from build123d import *

# Parameters (mm, degrees)
F0_W         = 34.925
F0_H         = 52.705
F1_DEPTH     = 9.7155
F2_W         = 25.781
F2_H         = 43.18
F2_H_2       = 40.005
F3_DEPTH     = 25.4
F4_R         = 8.255
F5_SIZE      = 0.8255
F6_R         = 1.5875
F7_DEPTH     = 25.4
F8_T1_DEPTH  = 34.1927991577
F9_SIZE      = 0.79375
F10_R        = 1.5875
F11_DEPTH    = 25.4
F13_R        = 7.493
F14_DEPTH    = 50.8
F15_T1_DEPTH = 13.2391086204
F15_T3_DEPTH = 13.2391086204
F16_W        = 2.54
F16_H        = 15.24
F17_DEPTH    = 25.4


# Not quite as in the source:
# - a fillet or chamfer that OpenCascade refuses, or shapes differently, is made with other operations: its cross-section is extruded or revolved along the edge and cut away or added
# - a feature names something its author has since deleted; it is built from what else it names


with BuildPart() as f1:
    # F0 (on Top) → F1 (new body)
    with BuildSketch(Plane.XY):
        with Locations((-17.4625, -26.3525)):
            Rectangle(F0_W, F0_H)
        with Locations((-17.4625, 26.3525)):
            Rectangle(F0_W, F0_H)
        Polygon((0, 52.705), (0, 0), (0, -52.705), (34.925, -52.705), (34.925, 0), (34.925, 52.705), align=None)
    extrude(amount=F1_DEPTH)

    # F2 (on face) → F3 (cut)
    with BuildSketch(Plane.XY.offset(9.7155)):
        with Locations((-12.8905, -21.59)):
            Rectangle(F2_W, F2_H)
        with Locations((-12.8905, 20.0025)):
            Rectangle(F2_W, F2_H_2)
        with Locations((12.8905, -21.59)):
            Rectangle(F2_W, F2_H)
        with Locations((12.8905, 20.0025)):
            Rectangle(F2_W, F2_H_2)
    extrude(amount=-F3_DEPTH, mode=Mode.SUBTRACT)

    # F4
    f4_edges = [f1.edges().sort_by_distance(p)[0] for p in [
        (-25.781, 40.005, 4.85775),
        (25.781, 40.005, 4.85775),
        (-25.781, -43.18, 4.85775),
        (25.781, -43.18, 4.85775),
    ]]
    fillet(f4_edges, radius=F4_R)

    # F5
    f5_edges = [f1.edges().sort_by_distance(p)[0] for p in [
        (-34.925, 0, 9.7155),
        (-25.781, -1.5875, 9.7155),
        (34.925, 0, 9.7155),
        (0, -52.705, 9.7155),
        (0, 52.705, 9.7155),
        (-34.925, 0, 0),
        (0, -52.705, 0),
        (34.925, 0, 0),
        (25.781, -1.5875, 0),
        (0, 52.705, 0),
        (-25.781, -1.5875, 0),
        (-23.363166, 37.587166, 0),
        (-23.363166, -40.762166, 0),
        (0, 40.005, 0),
        (0, -43.18, 0),
        (23.363166, 37.587166, 0),
        (23.363166, -40.762166, 0),
        (-23.363166, 37.587166, 9.7155),
        (-23.363166, -40.762166, 9.7155),
        (0, 40.005, 9.7155),
        (0, -43.18, 9.7155),
        (23.363166, 37.587166, 9.7155),
        (23.363166, -40.762166, 9.7155),
        (25.781, -1.5875, 9.7155),
    ]]
    chamfer(f5_edges, length=F5_SIZE)

    # F6 (on face) → F7 (cut)
    with BuildSketch(Plane(origin=(0, 52.705, 0), x_dir=(-1, 0, 0), z_dir=(0, 1, 0))):
        with Locations((-16.51, 4.7625)):
            Circle(F6_R)
        with Locations((16.51, 4.7625)):
            Circle(F6_R)
    extrude(amount=-F7_DEPTH, mode=Mode.SUBTRACT)

    # F8: chamfer of 5.08 on 2 edges, made by hand

    # F8_s2 → F8_t1 (cut)
    with BuildSketch(Plane.XY.offset(-12.2386495789)):
        Polygon((-34.925, -47.625), (-29.845, -52.705), (-34.925, -52.705), align=None)
        Polygon((29.845, -52.705), (34.925, -47.625), (34.925, -52.705), align=None)
    extrude(amount=F8_T1_DEPTH, mode=Mode.SUBTRACT)

    # F9
    f9_edges = [f1.edges().sort_by_distance(p)[0] for p in [
        (-32.385, -50.165, 0),
        (32.385, -50.165, 0),
        (32.385, -50.165, 9.7155),
        (-32.385, -50.165, 9.7155),
    ]]
    chamfer(f9_edges, length=F9_SIZE)

    # F10 (on face) → F11 (cut)
    with BuildSketch(Plane.XZ.offset(52.705)):
        with Locations((0, 4.7625)):
            Circle(F10_R)
    extrude(amount=-F11_DEPTH, mode=Mode.SUBTRACT)

    # F13 (on face) + F2 (on face) → F14 (cut)
    with BuildSketch(Plane(origin=(8.524875, 0, -14.7655166282), x_dir=(0.8660254038, 0, 0.5), z_dir=(0.5, 0, -0.8660254038))):
        with Locations((2.460086914, -52.705)):
            Circle(F13_R)
    with BuildSketch(Plane.XY.offset(9.7155)):
        with Locations((-12.8905, -21.59)):
            Rectangle(F2_W, F2_H)
        with Locations((-12.8905, 20.0025)):
            Rectangle(F2_W, F2_H_2)
        with Locations((12.8905, -21.59)):
            Rectangle(F2_W, F2_H)
        with Locations((12.8905, 20.0025)):
            Rectangle(F2_W, F2_H_2)
    extrude(amount=-F14_DEPTH, dir=(0.5, 0, -0.8660254038), mode=Mode.SUBTRACT)

    # F15: chamfer of 0.8001 on 2 edges, made by hand

    # F15_s2 → F15_t1 (cut)
    with BuildSketch(Plane(origin=(3.3783625895, 0, -5.8514956514), x_dir=(0, 1, 0), z_dir=(-0.5, 0, 0.8660254038))):
        with BuildLine():
            Line((52.705, -10.7145007393), (51.9820918836, -9.9181330962))
            ThreePointArc((51.9820918836, -9.9181330962), (52.3317918419, -9.9437868459), (52.705, -9.953086914))
            Line((52.705, -9.953086914), (52.705, -10.7145007393))
        make_face()
    extrude(amount=F15_T1_DEPTH, mode=Mode.SUBTRACT)

    # F15_s4 → F15_t3 (cut)
    with BuildSketch(Plane(origin=(-7.5672772878, 0, 13.1069087374), x_dir=(0, 1, 0), z_dir=(0.5, 0, -0.8660254038))):
        with BuildLine():
            Line((52.705, -5.7943269113), (51.9820918836, -4.9979592682))
            ThreePointArc((51.9820918836, -4.9979592682), (52.3317918419, -5.0236130179), (52.705, -5.032913086))
            Line((52.705, -5.032913086), (52.705, -5.7943269113))
        make_face()
    extrude(amount=F15_T3_DEPTH, mode=Mode.SUBTRACT)

    # F16 (on face) → F17 (cut)
    with BuildSketch(Plane.XZ.offset(-40.005)):
        with Locations((0, 5.08)):
            Rectangle(F16_W, F16_H)
    extrude(amount=-F17_DEPTH, mode=Mode.SUBTRACT)


solid = f1.part
Model file for the job. Use its own axes, mm. A direction names the side the tool comes from. Give positions to 0.01 mm unless a question says otherwise; leave off trailing zeros. Order: outer loops, then holes, each group sorted by start corner. A loop starts at its lowest first (then second) coordinate and runs counter-clockwise, first axis right, second up. Notation, with made-up numbers: M 39.5,43.25 L 98.5,43.25 A21 ccw 98.5,78.25 Z; hole C -39,0 d9. An arc over 180 degrees is marked long. Write item = value, one per line.
Q1. Tool access for faces 1 (the flat face through (-8.964, 52.349, 4.722)), 2 (the cylindrical face through (-23.3, 37.65, 4.8)), 3 (the flat face through (1.27, 43, 5)): list every direction of +Z, -Z, +X, -X, +Y, -Y with a clear straight run to the whole face (end or side of a thin tool).
Derived:
face_1 = +Z, +Y
face_2 = +Z, -Z
face_3 = +Z, -Z, +Y
Q2. Cut at B-B, the plane y = -4.5. List the corners of the cut face in (x, z) (1 decimal).
Derived:
outline = M -34.9,0.8 L -34.1,0 L -26.6,0 L -25.8,0.8 L -25.8,8.9 L -26.6,9.7 L -34.1,9.7 L -34.9,8.9 Z; M 25.8,0.8 L 26.6,0 L 34.1,0 L 34.9,0.8 L 34.9,8.9 L 34.1,9.7 L 26.6,9.7 L 25.8,8.9 Z
Q3. Cut at C-C, the plane x = 16. List the corners of the cut face in (y, z) (1 decimal).
Derived:
outline = M -52.7,0.8 L -51.9,0 L -44,0 L -43.2,0.8 L -43.2,8.9 L -44,9.7 L -51.9,9.7 L -52.7,8.9 Z; M 40,0.8 L 40.8,0 L 51.9,0 L 52.7,0.8 L 52.7,3.3 L 40,3.3 Z; M 40,6.3 L 52.7,6.3 L 52.7,8.9 L 51.9,9.7 L 40.8,9.7 L 40,8.9 Z
Q4. Two-plate mould, pull along Y, no slides. Class faces 4 (the cylindrical face through (6.5, 47.71, 4.83)), 5 (the conical face through (23.53, 37.62, 9.03)), 6 (the flat face through (-1.27, 43, 5)): pulls with the +Y half, pulls with the -Y half, needs draft (parallel to the pull), parting line crosses it, or undercut.
Derived:
face_4 = pulls with the +Y half
face_5 = undercut
face_6 = needs draft
Q5. Drill centre lines: line 1 (Y direction, x = -11, z = 2.75) (3 decimals); line 2 (X direction, y = -13.5, z = 2.5) (3 decimals); line 3 (Y direction, x = -1.5, z = 8) (3 decimals). Where is each one in solid material? Low to high. Write a range as [from, to].
Derived:
line_1 = [-52.705, -43.18], [40.005, 52.705]
line_2 = [-34.925, -25.781], [25.781, 34.925]
line_3 = [-52.705, -43.18], [40.005, 45.216]
Q6. Flat gauge pins, fed straight in: pin 1 (10 mm diameter, centred on x = 16.5, y = -30.5, fed in from -Z); pin 2 (4 mm diameter, centred on x = 0, z = 4.76, fed in from +Y). Where does each tip first touch, or does it go through?
Derived:
pin_1 = through
pin_2 = 45.51
